Here's how the part is built. I have some questions about the finished solid (model axes, mm). Give positions to 0.01 mm unless a question says otherwise; leave off trailing zeros. Loops run counter-clockwise (first coordinate to the right, second up) from the corner with the lowest first, then second, coordinate; pieces in that order, holes last. Notation, with made-up numbers: (-12.75, 77.25) - (2.25, 77.25) arc R17 cw to (2.25, 109.25) - close; hole circle Ø1 at (-10.75, 27). An arc over 180 degrees is marked (long way). Use a Markdown table: item, result.
Autodesk Inventor part; units mm, degrees
ref_plane "YZ Plane" through (0, 0, 0) normal (1, 0, 0) x (0, 1, 0)
ref_plane "XZ Plane" through (0, 0, 0) normal (0, 1, 0) x (-1, 0, 0)
ref_plane "XY Plane" through (0, 0, 0) normal (0, 0, 1) x (1, 0, 0)
sketch "Sketch1" plane through (0, 0, 0) normal (0, 1, 0) x (-1, 0, 0)
  line L0 (0, 0) -> (0, -1000)
  line L1 (0, -1000) -> (150, -1000)
  line L2 (150, -1000) -> (150, 0)
  circle A0 centre (150, 0) radius 150
  circle A1 centre (150, -1000) radius 150
  line L3 (300, 0) -> (300, -1000)
  circle A2 centre (150, 0) radius 75
  circle A3 centre (150, -1000) radius 75
  dimension "d0" = 1000
  dimension "d1" = 150
  dimension "d2" = 1000
  dimension "d3" = 150
  dimension "d4" = 150
extrude "Extrusion1" add sketch "Sketch1" along normal blind 300 contours A0 L2 A1 L0 | A0 | A1 L2 A3 L1 | L1 A3 L2 A1 | L3 A1 L2 A0
equation "\"BendRadius\" = Thickness"
equation "\"BendReliefWidth\" = Thickness"
equation "\"BendReliefDepth\" = 0.5 * Thickness"
equation "\"CornerReliefSize\" = 4 * Thickness"
equation "\"MinimumRemnant\" = 2 * Thickness"
equation "\"TransitionRadius\" = BendRadius"
equation "\"JacobiRadiusSize\" = BendRadius"
equation "\"GapSize\" = Thickness"
properties part number "Middle v2" material "Steel"
(1) Suppose I cut it at C-C on x = -204.5. Write out the boundary of the cut face in (y, z), plus the area to 3 significant figures.
A:
| item | result |
|---|---|
| outline | (0, -1139.75) - (300, -1139.75) - (300, -1051.52) - (0, -1051.52) - close; (0, -948.48) - (300, -948.48) - (300, -51.52) - (0, -51.52) - close; (0, 51.52) - (300, 51.52) - (300, 139.75) - (0, 139.75) - close |
| area | 322,000 mm2 |
(2) Suppose I cut it at B-B on y = 239.5. Write out the boundary of the cut face in (x, z).
A:
| item | result |
|---|---|
| outline | (-300, -1000) arc R150 ccw to (0, -1000) - (0, 0) arc R150 ccw to (-300, 0) - close; hole circle Ø150 at (-150, -1000); hole circle Ø150 at (-150, 0) |
(3) Will these pins go through, and if not, where does the flat tip stop? pin 1 (12 mm diameter, centred on x = -94, y = 228.5, fed in from -Z); pin 2 (5 mm diameter, centred on x = -260, y = 36.5, fed in from +Z); pin 3 (1.5 mm diameter, centred on x = -144, y = 47, fed in from -Z).
A:
| item | result |
|---|---|
| pin 1 | z = -1141.42 |
| pin 2 | z = 104.61 |
| pin 3 | z = -1149.91 |
(4) Suppose I cut it at A-A on x = -150. Write out the boundary of the cut face in (y, z), plus the area to 3 significant figures.
A:
| item | result |
|---|---|
| outline | (0, -1150) - (300, -1150) - (300, -1075) - (0, -1075) - close; (0, -925) - (300, -925) - (300, -75) - (0, -75) - close; (0, 75) - (300, 75) - (300, 150) - (0, 150) - close |
| area | 300,000 mm2 |
(5) If I drill on line 1 (Z direction, x = -150, y = 65); line 2 (X direction, y = 181, z = 0); line 3 (Z direction, x = -113, y = 271), over which ranges is the centre line in solid material (lowest first)?
A:
| item | result |
|---|---|
| line 1 | -1150 to -1075, -925 to -75, 75 to 150 |
| line 2 | -300 to -225, -75 to 0 |
| line 3 | -1145.37 to -1065.24, -934.76 to -65.24, 65.24 to 145.37 |
(6) We'd pull the mould along X, two halves only. Please class faces 1 (the face through (-148, 300, -491)), 2 (the face through (-153.298, 147.9, -1149.964)), 3 (the face through (-221.537, 147.9, -22.528)), 4 (the face through (-300, 148, -493)): pulls with the +X half, pulls with the -X half, needs draft (parallel to the pull), parting line crosses it, or undercut.
A:
| item | result |
|---|---|
| face 1 | needs draft |
| face 2 | parting line crosses it |
| face 3 | undercut |
| face 4 | pulls with the -X half |
